Work out the finished part from the listing and answer in its coordinate system (mm). A direction names the side the tool comes from. Coordinates: 2 decimals unless noted, no trailing zeros. Order: outer loops, then holes, each group sorted by start corner. A loop starts at its lowest first (then second) coordinate and runs counter-clockwise, first axis right, second up. Notation, with made-up numbers: (-6, 13.5) -> (20, 13.5) arc R27 ccw to (20, 31.5) -> close; hole circle Ø10 at (37.5, 11). An arc over 180 degrees is marked (long way). Write item = value, one per line. Start each with the question number.
Q1. Straight lines are drawn through the part: L1, parallel to Y at x = 0, z = 15.8; L2, parallel to X at y = -8, z = 10.5; L3, parallel to Y at x = -5.5, z = 1.25. For each, find the intervals that lie inside material, in ascending order. Write a range as from..to.
Q2. The part is cut by section A-A, the plane y = 6. Determine the outline of the cut face in (x, z).
Q3. Which of the six approach directions +Z, -Z, +X, -X, +Y, -Y give full straight-line access (tool end or side, diameter ignored) to faces 1 (the flat face through (8.069, 2.577, 7.605)), 2 (the flat face through (-8, 1, 15)), 3 (the flat face through (4.11, 2.85, 7.6))?
Q4. Flat-ended cylindrical pins translate along their axes: pin 1 (2 mm diameter, centred on x = 8, z = 11.5, fed in from +Y); pin 2 (4.5 mm diameter, centred on x = 0, y = 0, fed in from +Z); pin 3 (5 mm diameter, centred on y = 6.5, z = 8, fed in from +X); pin 4 (3 mm diameter, centred on x = 0, y = 0, fed in from +Z). Find the tip coordinate at first contact, or state that the pin passes through.
```python
from build123d import *

# Parameters (mm, degrees)
SKETCH_R           = 11.75
PAD_DEPTH          = 15
SKETCH001_R        = 1.7
POCKET_DEPTH       = 15.001
POCKET001_DEPTH    = 87.925619
POLARPATTERN_COUNT = 13
CHAMFER_SIZE       = 1
CHAMFER001_SIZE    = 1
FILLET_R           = 1
FILLET001_R        = 1
SKETCH003_R        = 11.75
PAD001_DEPTH       = 2
PAD001_FACE6_R     = 2.7
POCKET002_DEPTH    = 5


with BuildPart() as part:
    # Sketch → Pad (new body)
    with BuildSketch(Plane.XY):
        Circle(SKETCH_R)
    extrude(amount=PAD_DEPTH)

    # Sketch001 (on Face3 of Pad) → Pocket (cut, through all)
    with BuildSketch(Plane.XY.offset(15)):
        Circle(SKETCH001_R)
    extrude(amount=-POCKET_DEPTH, mode=Mode.SUBTRACT)

    # Sketch002 (on Face3 of Pocket) → Pocket001 (cut, through all)
    with BuildSketch(Plane.XY.offset(15)):
        Polygon((-1, 5), (1, 5), (2.389189, 12.878461), (-2.389183, 12.878462), align=None)
    pocket001 = extrude(amount=-POCKET001_DEPTH, mode=Mode.SUBTRACT)

    # PolarPattern: Pocket001 ×13 about axis
    polarpattern_axis = Axis((0, 0, 15), (0, 0, 1))
    for i in range(1, POLARPATTERN_COUNT):
        add(pocket001.rotate(polarpattern_axis, i * 360 / POLARPATTERN_COUNT), mode=Mode.SUBTRACT)

    # Chamfer
    chamfer_edges = [part.edges().sort_by_distance(p)[0] for p in [
        (-1.7, 0, 0),
    ]]
    chamfer(chamfer_edges, length=CHAMFER_SIZE)

    # Chamfer001
    chamfer001_edges = [part.edges().sort_by_distance(p)[0] for p in [
        (-1.7, 0, 15),
    ]]
    chamfer(chamfer001_edges, length=CHAMFER001_SIZE)

    # Fillet
    fillet_edges = [part.edges().sort_by_distance(p)[0] for p in [
        (-1.7, 0, 1),
    ]]
    fillet(fillet_edges, radius=FILLET_R)

    # Fillet001
    fillet001_edges = [part.edges().sort_by_distance(p)[0] for p in [
        (-1.7, 0, 14),
    ]]
    fillet(fillet001_edges, radius=FILLET001_R)

    # Sketch003 (on Face55 of PolarPattern) → Pad001 (join)
    with BuildSketch(Plane.XY.offset(15)):
        Circle(SKETCH003_R)
    extrude(amount=PAD001_DEPTH)

    # Pad001 Face6 → Pocket002 (cut)
    with BuildSketch(Plane(origin=(0, 0, 15), x_dir=(0, -1, 0), z_dir=(0, 0, -1))):
        Circle(PAD001_FACE6_R)
    extrude(amount=-POCKET002_DEPTH, mode=Mode.SUBTRACT)


solid = part.part
```
Model answer:
q1.L1 = -11.75..-2.7, 2.7..11.75
q1.L2 = -4.77..-3.66, -0.42..0.42, 3.66..4.77
q1.L3 = -10.38..-9.18, -4.22..-3.41, -0.93..-0.41, 1.8..2.39, 5.59..6.93
q2.outline = (-10.1, 15) -> (-5.92, 15) -> (-5.92, 0) -> (-4.78, 0) -> (-4.78, 15) -> (-1.79, 15) -> (-1.79, 0) -> (-1.18, 0) -> (-1.18, 15) -> (1.18, 15) -> (1.18, 0) -> (1.79, 0) -> (1.79, 15) -> (4.78, 15) -> (4.78, 0) -> (5.92, 0) -> (5.92, 15) -> (10.1, 15) -> (10.1, 17) -> (-10.1, 17) -> close
q3.face_1 = -Z, +X
q3.face_2 = -Z, -X
q3.face_3 = -Z
q4.pin_1 = 9.23
q4.pin_2 = 14.55
q4.pin_3 = 11.05
q4.pin_4 = through
